Print and shaded views of the part. All mm, measured from the part's lowest x, y and z. A direction names the side the tool comes from. Coordinates: 2 decimals unless noted, no trailing zeros. Loops run counter-clockwise (first coordinate to the right, second up) from the corner with the lowest first, then second, coordinate; pieces in that order, holes last.
1) Which spindle directions (+Z, -Z, +X, -X, +Y, -Y) get a long thin tool onto all of the face, cutting with end or side? Do the marked faces 1 and 2. Say none if no direction does.
2) Saw through at B-B, the plane x = 12.7. Write the cut outline in (y, z), and give its area (3 significant figures).
3) Saw through at D-D, the plane y = 2.1. Write the cut outline in (x, z), and give its area (3 significant figures).
4) Saw through at C-C, the plane y = 4.1. Write the cut outline in (x, z), and give its area (3 significant figures).
5) Wall check: line 1 along X through (y, z) = (3.4, 12.7); line 2 along X through (y, z) = (1.7, 12.7); line 3 along Z through (x, y) = (6.5, 1.75). Give the ranges that are in metal, low to high.
6) Two-plate mould, pull along Z, no slides. Class the marked faces 3, 4 and 5: +Z half, -Z half, draft (parallel to the pull), parting line (faces both ways), or undercut.
7) Saw through at A-A, the plane z = 12.7. Write the cut outline in (x, y).
8) Pin check, flat tips, straight feed: pin 1 Ø2 at (y, z) = (1, 11) entering from -X; pin 2 Ø1.5 at (y, z) = (2, 4.5) entering from +X; pin 3 Ø2 at (x, z) = (4, 3) entering from +Y; pin 4 Ø2 at (x, y) = (20, 4.5) entering from +Z. Stop position of each tip, or through.
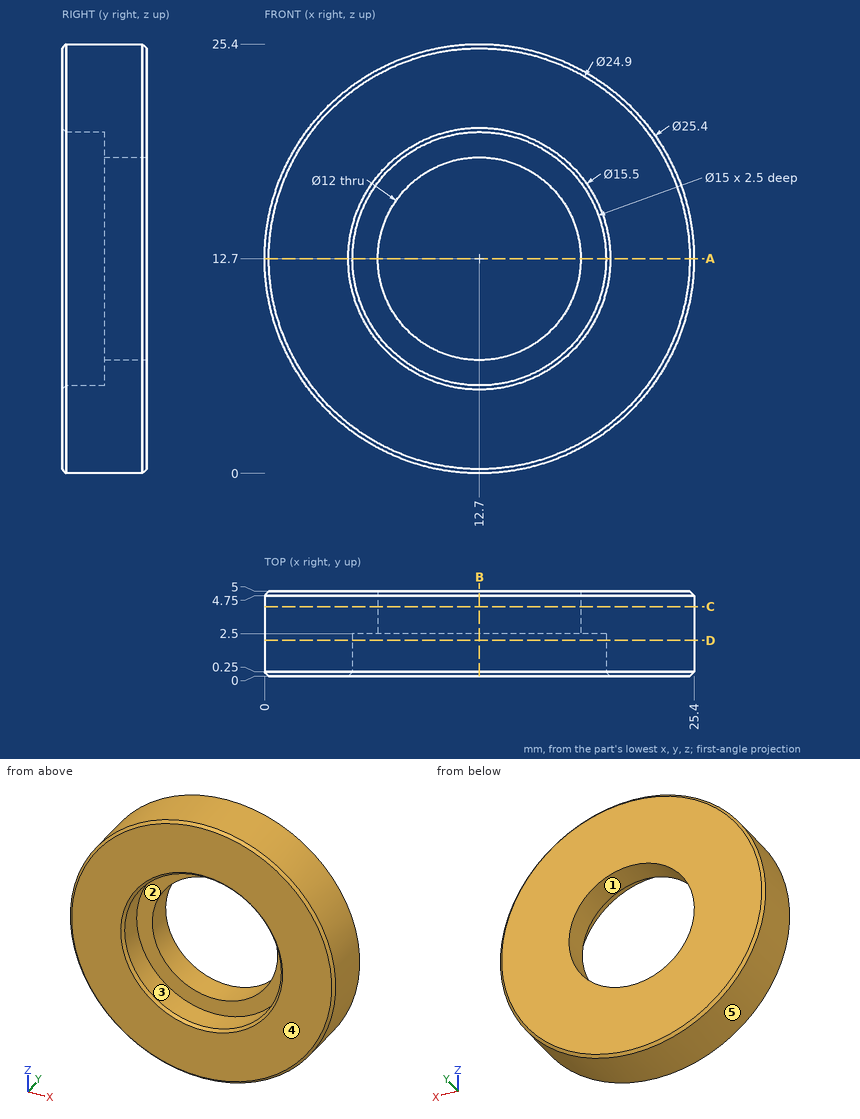
Data:
1. face 1: +Y, -Y
1. face 2: -Y
2. outline: (0, 0.25) - (0.25, 0) - (4.75, 0) - (5, 0.25) - (5, 6.7) - (2.5, 6.7) - (2.5, 5.2) - (0.25, 5.2) - (0, 4.95) - close; (0, 20.45) - (0.25, 20.2) - (2.5, 20.2) - (2.5, 18.7) - (5, 18.7) - (5, 25.15) - (4.75, 25.4) - (0.25, 25.4) - (0, 25.15) - close
2. area: 59.3 mm2
3. outline: circle Ø25.4 at (12.7, 12.7); hole circle Ø15 at (12.7, 12.7)
3. area: 330 mm2
4. outline: circle Ø25.4 at (12.7, 12.7); hole circle Ø12 at (12.7, 12.7)
4. area: 394 mm2
5. line 1: x = 0 to 6.7, 18.7 to 25.4
5. line 2: x = 0 to 5.2, 20.2 to 25.4
5. line 3: z = 1.62 to 8.48, 16.92 to 23.78
6. face 3: undercut
6. face 4: draft
6. face 5: parting line
7. outline: (0, 0.25) - (0.25, 0) - (4.95, 0) - (5.2, 0.25) - (5.2, 2.5) - (6.7, 2.5) - (6.7, 5) - (0.25, 5) - (0, 4.75) - close; (18.7, 2.5) - (20.2, 2.5) - (20.2, 0.25) - (20.45, 0) - (25.15, 0) - (25.4, 0.25) - (25.4, 4.75) - (25.15, 5) - (18.7, 5) - close
8. pin 1: stops at x = 0.02
8. pin 2: stops at x = 22.99
8. pin 3: stops at y = 5
8. pin 4: stops at z = 23.73
